Check sheet for the modelled part. Datum: model origin and axes. Units: mm. Round coordinates to 2 decimals unless told otherwise and drop trailing zeros. Write each loop counter-clockwise with the first axis right and the second up, starting at its lowest first coordinate (ties: lowest second). Pieces come first, ordered by that corner, then holes. Notation, with made-up numbers: (72, 69.25) -> (100, 69.25) arc R23 cw to (100, 93.25) -> close; hole circle Ø4 at (51.25, 28). An arc over 180 degrees is marked (long way). One line per item, written item: value.
from build123d import *

# Parameters (mm, degrees)
CYLINDER001_R           = 1.5
CYLINDER001_DEPTH       = 44
CYLINDER001_PITCH_ANGLE = 90
CYLINDER_R              = 2.5
CYLINDER_DEPTH          = 40
CYLINDER_PITCH_ANGLE    = 90


with BuildPart() as cilindro001:
    # Cylinder001 → Cylinder001 (new body)
    with BuildSketch(Plane.XY):
        Circle(CYLINDER001_R)
    extrude(amount=CYLINDER001_DEPTH)


with BuildPart() as cilindro001_1:
    # Cylinder001 pitch: moved
    add(cilindro001.part.rotate(Axis((0, 0, 0), (0, 1, 0)), CYLINDER001_PITCH_ANGLE))


with BuildPart() as cilindro001_2:
    # Cylinder001 placement: moved
    add(cilindro001_1.part.moved(Location((-2, 0, 0))))


with BuildPart() as soporte1:
    # Cylinder → Cylinder (new body)
    with BuildSketch(Plane.XY):
        Circle(CYLINDER_R)
    extrude(amount=CYLINDER_DEPTH)


with BuildPart() as soporte1_1:
    # Cylinder pitch: moved
    add(soporte1.part.rotate(Axis((0, 0, 0), (0, 1, 0)), CYLINDER_PITCH_ANGLE))


with BuildPart() as soporte1_2:
    # Cylinder placement: moved
    add(soporte1_1.part)

    # Cut: cut Cilindro001
    add(cilindro001_2.part, mode=Mode.SUBTRACT)


with BuildPart() as soporte1_3:
    # Cut placement: moved
    add(soporte1_2.part.moved(Location((235, 175.5, 291))))


solid = soporte1_3.part
Item 1: Sectioned sample at D-D on z = 289.1. Enter the section's corners in (x, y), and give its area (3 significant figures).
Answer:
outline: (235, 173.88) -> (275, 173.88) -> (275, 177.12) -> (235, 177.12) -> close
area: 130 mm^2
Item 2: Sectioned sample at B-B on y = 175.5. Enter the section's corners in (x, z).
Answer:
outline: (235, 288.5) -> (275, 288.5) -> (275, 289.5) -> (235, 289.5) -> close; (235, 292.5) -> (275, 292.5) -> (275, 293.5) -> (235, 293.5) -> close
Item 3: Mould release check, pull along Z, two halves, no side actions. Record for faces 1 (the cylindrical face through (254.72, 177.61, 289.66)), 2 (the flat face through (275, 174, 290)), 3 (the cylindrical face through (254.72, 175.95, 289.57)): pulls with the +Z half, pulls with the -Z half, needs draft (parallel to the pull), parting line crosses it, or undercut.
Answer:
face 1: parting line crosses it
face 2: needs draft
face 3: undercut
Item 4: Sectioned sample at C-C on x = 272. Enter the section's corners in (y, z).
Answer:
outline: circle Ø5 at (175.5, 291); hole circle Ø3 at (175.5, 291)
Item 5: Sectioned sample at A-A on z = 291. Enter the section's corners in (x, y), and give its area (3 significant figures).
Answer:
outline: (235, 173) -> (275, 173) -> (275, 174) -> (235, 174) -> close; (235, 177) -> (275, 177) -> (275, 178) -> (235, 178) -> close
area: 80.0 mm^2
Item 6: Depth check by flat-ended pin: P1, Ø2, axis at x = 268.5, z = 292, coming from the -Y side; P2, Ø2.5, axis at y = 175.5, z = 291, coming from the +X side. Enter the tip coordinate at first touch or a pass-through.
Answer:
P1: stops at y = 173
P2: passes through
Item 7: Thickness scan on line 1 (Z direction, x = 247.5, y = 175.5); line 2 (Y direction, x = 258, z = 291); line 3 (Z direction, x = 264.5, y = 174.4) (3 decimals). Record the ranges inside material, lowest first.
Answer:
line 1: z = 288.5 to 289.5, 292.5 to 293.5
line 2: y = 173 to 174, 177 to 178
line 3: z = 288.755 to 289.98, 292.02 to 293.245
